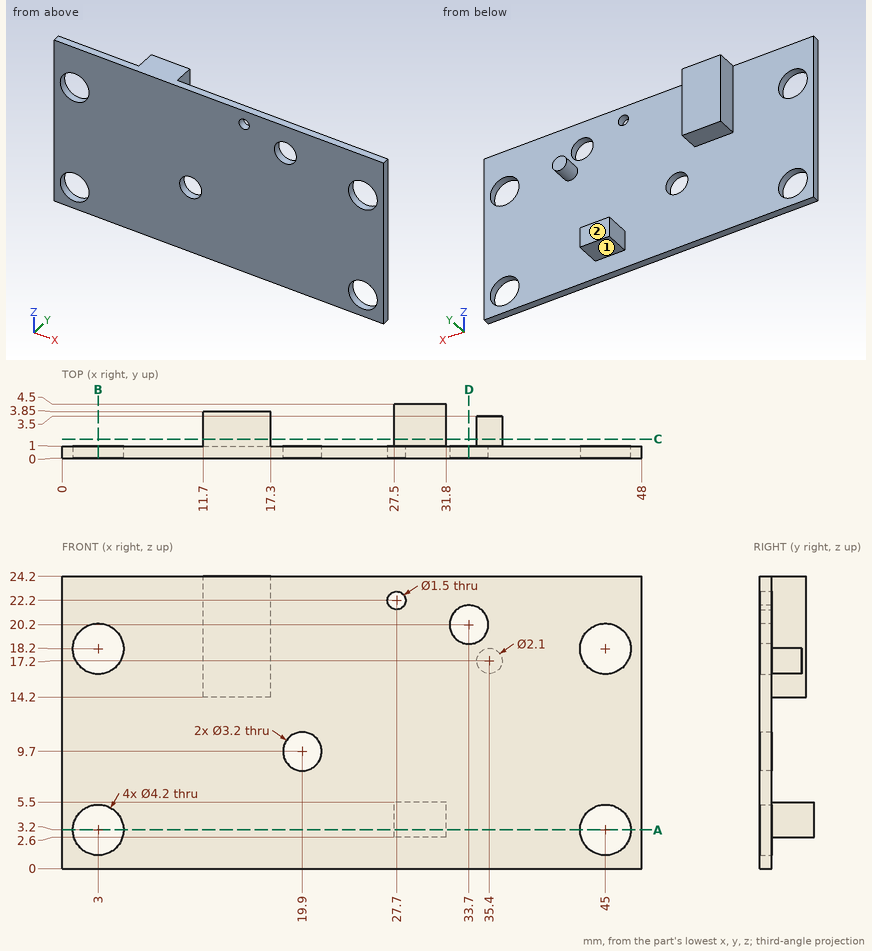
Study the drawing (mm; zero at the part's minimum x, y, z) and answer. A direction names the side the tool comes from. Round coordinates to 2 decimals unless told otherwise and drop trailing zeros. Write each loop counter-clockwise with the first axis right and the second up, starting at its lowest first coordinate (ties: lowest second). Pieces come first, ordered by that corner, then holes.
1) Which of the six approach directions +Z, -Z, +X, -X, +Y, -Y give full straight-line access (tool end or side, diameter ignored) to the marked faces 1 and 2?
2) A cutting plane is placed at A-A on z = 3.2. Determine the outline of the cut face in (x, y), and give its area (4 significant figures).
3) Consider probe 1 along Z at (x, y) = (3, 0.5); probe 2 along X at (y, z) = (0.4, 3); probe 3 along Z at (x, y) = (27.7, 0.35). Determine where each line is inside the solid, lowest interval first.
4) A cutting plane is placed at C-C on y = 1.6. Determine the outline of the cut face in (x, z).
5) A cutting plane is placed at B-B on x = 3. Determine the outline of the cut face in (y, z).
6) Flat-ended cylindrical pins translate along their axes: P1, Ø2.5, axis at x = 45, z = 18.2, coming from the -Y side; P2, Ø2.5, axis at y = 2, z = 17, coming from the -X side; P3, Ø12, axis at x = 14.5, z = 15, coming from the +Y side; P4, Ø6.5, axis at x = 45, z = 3.2, coming from the +Y side. Find the tip coordinate at first contact, or state that the pin passes through.
7) A cutting plane is placed at D-D on x = 33.7. Determine the outline of the cut face in (y, z).
Entries:
1. face 1: -Z, +X, -X, +Y
1. face 2: +Z, -Z, +X, -X, +Y
2. outline: (0, 0) - (0.9, 0) - (0.9, 1) - (0, 1) - close; (5.1, 0) - (42.9, 0) - (42.9, 1) - (31.8, 1) - (31.8, 4.5) - (27.5, 4.5) - (27.5, 1) - (5.1, 1) - close; (47.1, 0) - (48, 0) - (48, 1) - (47.1, 1) - close
2. area: 54.65 mm2
3. probe 1: z = 0 to 1.1, 5.3 to 16.1, 20.3 to 24.2
3. probe 2: x = 0 to 0.91, 5.09 to 42.91, 47.09 to 48
3. probe 3: z = 0 to 21.45, 22.95 to 24.2
4. outline: (11.7, 14.2) - (17.3, 14.2) - (17.3, 24.2) - (11.7, 24.2) - close; (27.5, 2.6) - (31.8, 2.6) - (31.8, 5.5) - (27.5, 5.5) - close; circle Ø2.1 at (35.4, 17.2)
5. outline: (0, 0) - (1, 0) - (1, 1.1) - (0, 1.1) - close; (0, 5.3) - (1, 5.3) - (1, 16.1) - (0, 16.1) - close; (0, 20.3) - (1, 20.3) - (1, 24.2) - (0, 24.2) - close
6. P1: passes through
6. P2: stops at x = 0
6. P3: stops at y = 3.85
6. P4: stops at y = 1
7. outline: (0, 0) - (1, 0) - (1, 18.6) - (0, 18.6) - close; (0, 21.8) - (1, 21.8) - (1, 24.2) - (0, 24.2) - close
